Read the model definition and answer for the solid it produces. Units are mm, in the model's axes. A direction names the side the tool comes from. Give positions to 0.01 mm unless a question says otherwise; leave off trailing zeros. Order: outer loops, then holes, each group sorted by start corner. A loop starts at its lowest first (then second) coordinate and runs counter-clockwise, first axis right, second up. Notation, with made-up numbers: (13.5, 8) - (69.5, 8) arc R12 ccw to (69.5, 18) - close; hole circle Ø11 at (-25.75, 4.5). An arc over 180 degrees is marked (long way). Return JSON: item names as keys, results as strings.
Autodesk Inventor part; units mm, degrees
ref_plane "YZ Plane" through (0, 0, 0) normal (1, 0, 0) x (0, 1, 0)
ref_plane "XZ Plane" through (0, 0, 0) normal (0, 1, 0) x (-1, 0, 0)
ref_plane "XY Plane" through (0, 0, 0) normal (0, 0, 1) x (1, 0, 0)
sketch "Sketch1" plane through (0, 0, 0) normal (1, 0, 0) x (0, 1, 0)
  line L0 (0, 0) -> (10, 0)
  line L1 (10, 0) -> (10, -10)
  line L2 (10, -10) -> (0, -10)
  line L3 (0, -10) -> (0, 0)
  dimension "d0" = 10
  dimension "d1" = 10
extrude "Extrusion1" add sketch "Sketch1" along normal blind 10
sketch "Sketch3" plane through (0, 0, 0) normal (-1, 0, 0) x (0, 0, 1)
  circle A0 centre (-5, 5) radius 1.5
  point P0 (0, 0)
extrude "Extrusion3" cut sketch "Sketch3" against normal blind 5
sketch "Sketch4" plane through (0, 0, 0) normal (0, 0, 1) x (1, 0, 0)
  line L0 (1.8731, 7.9408) -> (4.4271, 7.9408) construction
  line L1 (4.4271, 7.9408) -> (4.4271, 4.8928) construction
  line L2 (4.4271, 4.8928) -> (1.8731, 4.8928) construction
  line L3 (1.8731, 4.8928) -> (1.8731, 7.9408) construction
  spline S0 degree 2 poles (7.0108, 6.9784) (6.7321, 6.9784) (6.1484, 7.0258) knots 0 0 0 1 1 1
  spline S1 degree 2 poles (6.1484, 7.0258) (5.5857, 7.0678) (5.2912, 7.0626) knots 0 0 0 1 1 1
  line L4 (5.2912, 7.0626) -> (5.023, 7.0626)
  spline S2 degree 2 poles (5.023, 7.0626) (5.0336, 6.542) (5.1229, 5.3693) knots 0 0 0 1 1 1
  spline S3 degree 2 poles (5.1229, 5.3693) (5.2071, 4.2808) (5.2071, 3.676) knots 0 0 0 1 1 1
  spline S4 degree 2 poles (5.2071, 3.676) (5.2071, 3.5445) (5.2597, 3.0082) (5.2597, 2.8714) knots 0 0 0 1 2 2 2
  spline S5 degree 2 poles (5.2597, 2.8714) (5.2597, 2.619) (5.1755, 2.4297) knots 0 0 0 1 1 1
  spline S6 degree 2 poles (5.1755, 2.4297) (5.0704, 2.1826) (4.8495, 2.1826) knots 0 0 0 1 1 1
  spline S7 degree 2 poles (4.8495, 2.1826) (4.697, 2.1826) (4.4551, 2.3929) (4.4551, 2.5612) knots 0 0 0 1 2 2 2
  spline S8 degree 2 poles (4.4551, 2.5612) (4.4551, 2.619) (4.4919, 2.8452) (4.4919, 2.8977) knots 0 0 0 1 2 2 2
  spline S9 degree 2 poles (4.4919, 2.8977) (4.4919, 3.087) (4.4446, 3.8233) (4.4446, 4.0126) knots 0 0 0 1 2 2 2
  spline S10 degree 2 poles (4.4446, 4.0126) (4.4446, 4.5542) (4.3552, 5.5323) knots 0 0 0 1 1 1
  spline S11 degree 2 poles (4.3552, 5.5323) (4.2658, 6.584) (4.2553, 7.0468) knots 0 0 0 1 1 1
  line L5 (4.2553, 7.0468) -> (3.9135, 7.0415)
  spline S12 degree 2 poles (3.9135, 7.0415) (3.0879, 7.0415) (2.6146, 7.1625) knots 0 0 0 1 1 1
  spline S13 degree 2 poles (2.6146, 7.1625) (2.3096, 7.2414) (2.3096, 7.5358) knots 0 0 0 1 1 1
  spline S14 degree 2 poles (2.3096, 7.5358) (2.3096, 7.6936) (2.4095, 7.8093) knots 0 0 0 1 1 1
  spline S15 degree 2 poles (2.4095, 7.8093) (2.5199, 7.9408) (2.6987, 7.9302) knots 0 0 0 1 1 1
  spline S16 degree 2 poles (2.6987, 7.9302) (2.8302, 7.925) (3.3035, 7.8619) knots 0 0 0 1 1 1
  spline S17 degree 2 poles (3.3035, 7.8619) (3.6768, 7.8146) (3.9135, 7.8146) knots 0 0 0 1 1 1
  spline S18 degree 2 poles (3.9135, 7.8146) (4.1396, 7.8146) (5.0598, 7.8356) (5.286, 7.8356) knots 0 0 0 1 2 2 2
  spline S19 degree 2 poles (5.286, 7.8356) (5.5752, 7.8356) (6.7163, 7.7514) (7.0108, 7.7514) knots 0 0 0 1 2 2 2
  spline S20 degree 2 poles (7.0108, 7.7514) (7.1686, 7.7514) (7.3894, 7.5306) (7.3894, 7.3623) knots 0 0 0 1 2 2 2
  spline S21 degree 2 poles (7.3894, 7.3623) (7.3894, 7.2045) (7.1686, 6.9784) (7.0108, 6.9784) knots 0 0 0 1 2 2 2
  point P0 (0, 0)
extrude "Extrusion4" cut sketch "Sketch4" against normal blind 2
properties part number "Thymine1"
Q1. Given pin 1 (3.5 mm diameter, centred on y = 5, z = -4.5, fed in from -X), flat-ended and moving along its own axis, determine where the tip first touches the part or whether it passes through.
Values:
{"pin 1": "stops at x = 0"}
Q2. For faces 5 (the flat face through (4, 5, 0)), 6 (the flat face through (5, 5, -5)), determine the directions among +Z, -Z, +X, -X, +Y, -Y from which every point of the face is accessible in a straight line to the end or side of a thin tool.
Values:
{"face 5": "+Z, +X, -X, +Y, -Y", "face 6": "-X"}
Q3. Consider L1, parallel to Y at x = 1.3, z = -5; L2, parallel to Z at x = 2.5, y = 4; L3, parallel to X at y = 5.25, z = -6. Determine where each line is inside the solid, lowest interval first.
Values:
{"L1": "y = 0 to 3.5, 6.5 to 10", "L2": "z = -10 to -6.12, -3.88 to 0", "L3": "x = 5 to 10"}
Q4. Determine the mould class of faces 1 (the cylindrical face through (2.5, 4.1, -6.2)), 2 (the flat face through (5, 5, -10)), 3 (the flat face through (5, 10, -5)), 4 (the flat face through (5, 0, -5)) for opening direction Y: released by +Y, released by -Y, zero draft, split by the parting line, or undercut.
Values:
{"face 1": "undercut", "face 2": "zero draft", "face 3": "released by +Y", "face 4": "released by -Y"}
Q5. A cutting plane is placed at A-A (x = 1). Write down the section's boundary in (y, z).
Values:
{"outline": "(0, -10) - (10, -10) - (10, 0) - (0, 0) - close; hole circle Ø3 at (5, -5)"}
Q6. A cutting plane is placed at B-B (z = -5). Write down the section's boundary in (x, y), and give its area (3 significant figures).
Values:
{"outline": "(0, 0) - (10, 0) - (10, 10) - (0, 10) - (0, 6.5) - (5, 6.5) - (5, 3.5) - (0, 3.5) - close", "area": "85.0 mm²"}
